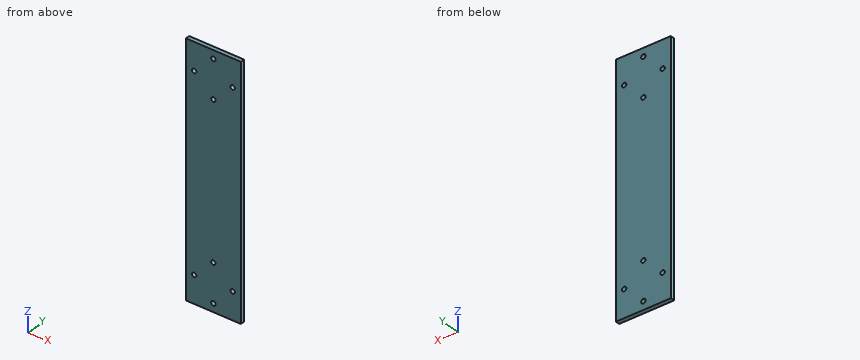
Autodesk Inventor part; units mm, degrees
ref_plane "YZ Plane" through (0, 0, 0) normal (1, 0, 0) x (0, 1, 0)
ref_plane "XZ Plane" through (0, 0, 0) normal (0, 1, 0) x (-1, 0, 0)
ref_plane "XY Plane" through (0, 0, 0) normal (0, 0, 1) x (1, 0, 0)
sketch "Sketch1" plane through (0, 0, 0) normal (0, 1, 0) x (-1, 0, 0)
  line L0 (10, -45) -> (-10, -45)
  line L1 (-10, -45) -> (-10, 45)
  line L2 (-10, 45) -> (10, 45)
  line L3 (10, 45) -> (10, -45)
  point P0 (0, 0)
  dimension "d0" = 20
  dimension "d1" = 90
  dimension "d2" = 45
  dimension "d3" = 10
extrude "Plate1" add sketch "Sketch1" along normal blind 1.5
sketch "Sketch2" plane through (0, 0, 0) normal (0, -1, 0) x (1, 0, 0)
  circle A0 centre (0, 42) radius 0.7835
  circle A1 centre (-7, 35) radius 0.7835
  circle A2 centre (0, 28) radius 0.7835
  circle A3 centre (7, 35) radius 0.7835
  circle A4 centre (0, -28) radius 0.7835
  circle A5 centre (-7, -35) radius 0.7835
  circle A6 centre (0, -42) radius 0.7835
  circle A7 centre (7, -35) radius 0.7835
  point P0 (0, 0)
hole "Hole1" at (0, 0, 42) at (-7, 0, 35) at (0, 0, 28) at (7, 0, 35) at (0, 0, -28) at (-7, 0, -35) at (0, 0, -42) at (7, 0, -35) direction (0, 1, 0) diameter 1.6 depth 1.5
equation "\"d10\" = Thickness"
equation "\"d4\" = Thickness"
equation "\"BendReliefWidth\" = Thickness"
equation "\"BendReliefDepth\" = 0.5 * Thickness"
equation "\"CornerReliefSize\" = 4 * Thickness"
equation "\"MinimumRemnant\" = 2 * Thickness"
equation "\"TransitionRadius\" = BendRadius"
equation "\"JacobiRadiusSize\" = BendRadius"
equation "\"GapSize\" = Thickness"
properties part number "axis_10_11-connector_frame" material "Aluminum 6061-AHC"
Geometry: final body of the model. Coordinates: model frame, mm. Coordinates: 2 decimals unless noted, no trailing zeros. Loops run counter-clockwise (first coordinate to the right, second up) from the corner with the lowest first, then second, coordinate; pieces in that order, holes last. Notation, with made-up numbers: M -33.5,-33.75 L -12.5,-33.75 A27 ccw -12.5,-7.75 Z; hole C 88,76 d4. An arc over 180 degrees is marked long. One line per item, written item: value. Start each with the question number.
1) Cut plane D-D (x = 0). Return loops of the section in (y, z).
2) Cut plane C-C (z = -35). Return loops of the section in (x, y), then the cut area to 3 significant figures.
3) Cut plane A-A (x = 7). Return loops of the section in (y, z).
4) Pin query (flat end, axial travel): P1, Ø2.5, axis at x = -7, z = -35, coming from the +Y side. Return the tip coordinate at first contact, or that it passes through.
5) Material intervals for L1, parallel to X at y = 0.3, z = 35; L2, parallel to Z at x = 0, y = 1; L3, parallel to Z at x = 7, y = 1.25, sorted ascending. Write a range as from..to.
6) Cut plane B-B (z = 42). Return loops of the section in (x, y), then the cut area to 3 significant figures.
Evaluation:
1. outline: M 0,-45 L 1.5,-45 L 1.5,-42.8 L 0,-42.8 Z; M 0,-41.2 L 1.5,-41.2 L 1.5,-28.8 L 0,-28.8 Z; M 0,-27.2 L 1.5,-27.2 L 1.5,27.2 L 0,27.2 Z; M 0,28.8 L 1.5,28.8 L 1.5,41.2 L 0,41.2 Z; M 0,42.8 L 1.5,42.8 L 1.5,45 L 0,45 Z
2. outline: M -10,0 L -7.8,0 L -7.8,1.5 L -10,1.5 Z; M -6.2,0 L 6.2,0 L 6.2,1.5 L -6.2,1.5 Z; M 7.8,0 L 10,0 L 10,1.5 L 7.8,1.5 Z
2. area: 25.2 mm^2
3. outline: M 0,-45 L 1.5,-45 L 1.5,-35.8 L 0,-35.8 Z; M 0,-34.2 L 1.5,-34.2 L 1.5,34.2 L 0,34.2 Z; M 0,35.8 L 1.5,35.8 L 1.5,45 L 0,45 Z
4. P1: y = 1.5
5. L1: -10..-7.8, -6.2..6.2, 7.8..10
5. L2: -45..-42.8, -41.2..-28.8, -27.2..27.2, 28.8..41.2, 42.8..45
5. L3: -45..-35.8, -34.2..34.2, 35.8..45
6. outline: M -10,0 L -0.8,0 L -0.8,1.5 L -10,1.5 Z; M 0.8,0 L 10,0 L 10,1.5 L 0.8,1.5 Z
6. area: 27.6 mm^2
